Can you work these out from the drawing? Everything is in mm from the part's minimum corner. Round coordinates to 2 decimals unless told otherwise and drop trailing zeros. Write each loop counter-clockwise with the first axis right and the second up, starting at its lowest first coordinate (ties: lowest second). Pieces come first, ordered by that corner, then holes. Notation, with made-up numbers: M 25.5,27.25 L 71.5,27.25 A23 cw 71.5,36.25 Z; hole C 74.25,73.25 d6. An arc over 180 degrees is marked long. Use one line per item in the form item = value. Start each with the question number.
Q1. I want a section at B-B on y = 52. List the corners of the cut face in (x, z) for me, and give its area (3 significant figures).
Q2. I want a section at D-D on y = 70.5. List the corners of the cut face in (x, z) for me, and give its area (3 significant figures).
Q3. I'm going to push flat-ended pins straight in: pin 1 Ø3 at (y, z) = (32.5, 13.5) entering from -X; pin 2 Ø3 at (x, z) = (34.5, 13) entering from +Y; pin 3 Ø4.5 at (y, z) = (34.5, 13) entering from +X; pin 4 Ø4 at (x, y) = (10, 16.5) entering from -Z. Where does each tip first touch, or does it pass through?
Q4. I need wall thicknesses on line 1 along X through (y, z) = (52, 12.5); line 2 along Y through (x, z) = (52.5, 13); line 3 along Z through (x, y) = (82, 14.5). Which ranges of each line are inside material? Lowest first, please. Write a range as from..to.
Q5. I want a section at A-A on z = 12.5. List the corners of the cut face in (x, y) for me, and give its area (3 significant figures).
Q6. I want a section at C-C on x = 13. List the corners of the cut face in (y, z) for me, and give its area (3 significant figures).
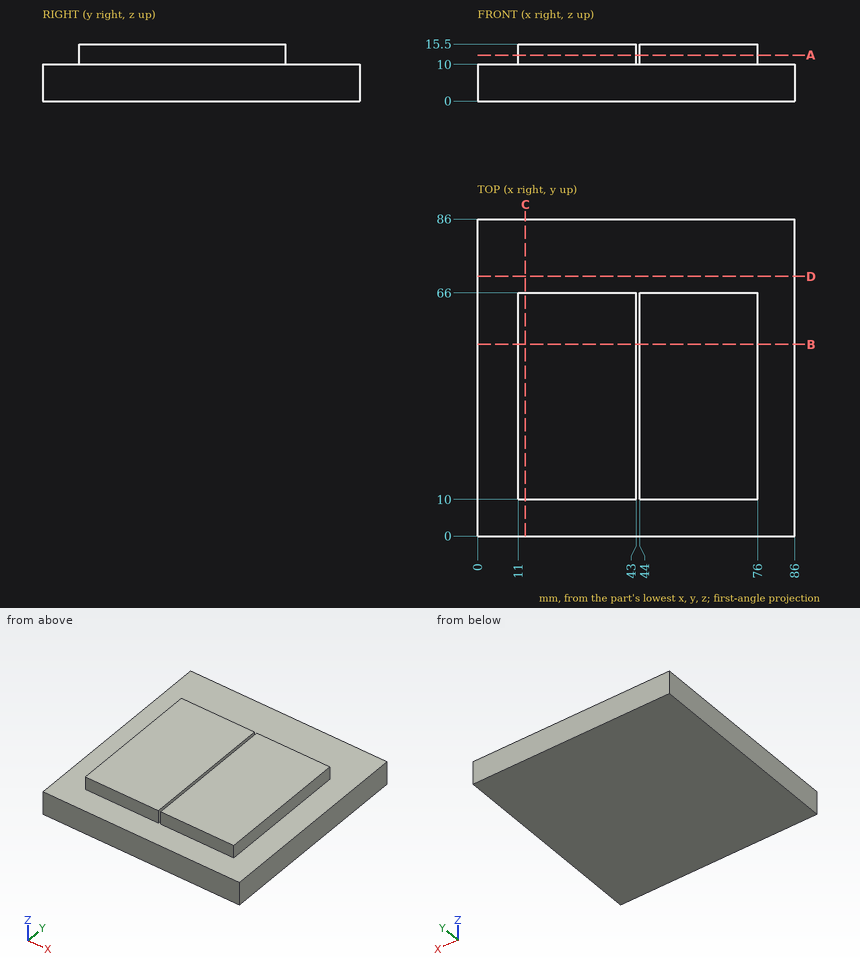
Reported:
q1.outline = M 0,0 L 86,0 L 86,10 L 76,10 L 76,15.5 L 44,15.5 L 44,10 L 43,10 L 43,15.5 L 11,15.5 L 11,10 L 0,10 Z
q1.area = 1,210 mm^2
q2.outline = M 0,0 L 86,0 L 86,10 L 0,10 Z
q2.area = 860 mm^2
q3.pin_1 = 11
q3.pin_2 = 66
q3.pin_3 = 76
q3.pin_4 = 0
q4.line_1 = 11..43, 44..76
q4.line_2 = 10..66
q4.line_3 = 0..10
q5.outline = M 11,10 L 43,10 L 43,66 L 11,66 Z; M 44,10 L 76,10 L 76,66 L 44,66 Z
q5.area = 3,580 mm^2
q6.outline = M 0,0 L 86,0 L 86,10 L 66,10 L 66,15.5 L 10,15.5 L 10,10 L 0,10 Z
q6.area = 1,170 mm^2
